Source: CAD feature listing. Evaluate the final solid. Frame: model axes, mm. Face numbers are marked on the shaded views. A direction names the side the tool comes from. Give positions to 0.01 mm unless a question says otherwise; leave off trailing zeros. Loops run counter-clockwise (first coordinate to the right, second up) from the corner with the lowest first, then second, coordinate; pieces in that order, holes last. Notation, with made-up numbers: (80.25, 10) -> (127.25, 10) arc R23 ccw to (127.25, 25) -> close; hole circle Ø2 at (37.5, -10). An arc over 180 degrees is marked (long way). Return JSON: item names as keys, results as strings. Group by question number.
(1) Cut plane A-A on x = -46. Return loops of the section in (y, z).
(2) Pin query (flat end, axial travel): pin 1 (6 mm diameter, centred on y = -50, z = 31, fed in from -X); pin 2 (4.5 mm diameter, centred on x = -46, y = -21.5, fed in from -Z); pin 3 (5 mm diameter, centred on x = -46, y = 15.7, fed in from -Z); pin 4 (1 mm diameter, centred on x = 95.5, z = 49, fed in from +Y). Return the tip coordinate at first contact, or that it passes through.
(3) Cut plane C-C on z = 63. Return loops of the section in (x, y).
(4) Cut plane B-B on y = 5.5. Return loops of the section in (x, z).
(5) Access query for the marked faces 1, 2 and 3. Directions: +Z, -Z, +X, -X, +Y, -Y. A direction counts if a zero-diameter tool reaches every point of the face in a straight line with its end or side. Return the directions, or none.
(6) Cut plane D-D on y = -52. Return loops of the section in (x, z) (3 decimals), then the cut area to 3 significant figures.
(7) Ray query, line 1 (Y direction, x = 0, z = 3.25); line 2 (Y direction, x = -32, z = 57); line 3 (X direction, y = -24, z = 35). Return the intervals inside material, ascending. Write a range as from..to.
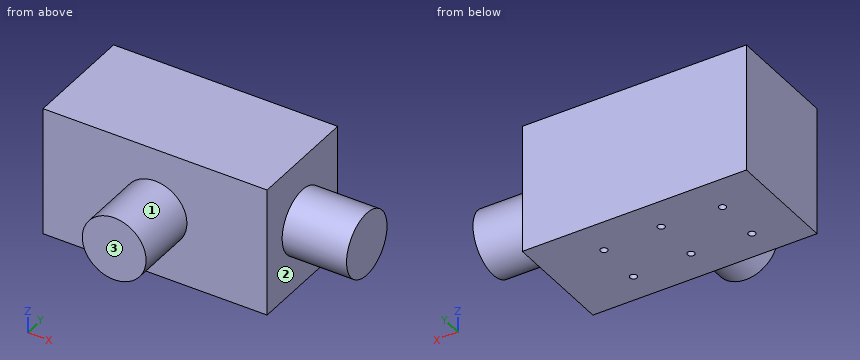
Autodesk Inventor part; units mm, degrees
ref_plane "YZ Plane" through (0, 0, 0) normal (1, 0, 0) x (0, 1, 0)
ref_plane "XZ Plane" through (0, 0, 0) normal (0, 1, 0) x (-1, 0, 0)
ref_plane "XY Plane" through (0, 0, 0) normal (0, 0, 1) x (1, 0, 0)
sketch "Sketch1" plane through (0, 0, 0) normal (0, 0, 1) x (1, 0, 0)
  line L0 (-13.5, 24) -> (13.5, 24) construction
  line L1 (13.5, 24) -> (13.5, -24) construction
  line L2 (13.5, -24) -> (-13.5, -24) construction
  line L3 (-13.5, -24) -> (-13.5, 24) construction
  line L4 (-13.5, 0) -> (13.5, 0) construction
  line L5 (0, -24) -> (0, 24) construction
  circle A0 centre (0, 18.3) radius 2.75
  circle A1 centre (0, -18.3) radius 2.75
  line L6 (-60, 21.2) -> (-32, 21.2) construction
  line L7 (-32, 21.2) -> (-32, -25.8) construction
  line L8 (-32, -25.8) -> (-60, -25.8) construction
  line L9 (-60, -25.8) -> (-60, 21.2) construction
  line L10 (-46, 21.2) -> (-46, -25.8) construction
  line L11 (-60, -2.3) -> (-32, -2.3) construction
  circle A2 centre (-46, 15.7) radius 2.75
  circle A3 centre (-46, -20.3) radius 2.75
  circle A4 centre (46, 15.7) radius 2.75
  circle A5 centre (46, -20.3) radius 2.75
  line L12 (-82, 43.2) -> (82, 43.2)
  line L13 (82, 43.2) -> (82, -43.2)
  line L14 (82, -43.2) -> (-82, -43.2)
  line L15 (-82, -43.2) -> (-82, 43.2)
  point P0 (0, 0)
  point P1 (0, 0)
  dimension "d0" = 27
  dimension "d1" = 48
  dimension "d2" = 5.5
  dimension "d3" = 36.6
  dimension "d4" = 28
  dimension "d5" = 47
  dimension "d7" = 2.3
  dimension "d8" = 46
  dimension "d9" = 5.5
  dimension "d10" = 36
  dimension "d11" = 22
  dimension "d19" = 43.2
extrude "Extrusion1" add sketch "Sketch1" along normal blind 10
sketch "Sketch3" plane through (0, 0, 10) normal (0, 0, 1) x (1, 0, 0)
  line L0 (-82, 43.2) -> (-82, -43.2)
  line L1 (-82, -43.2) -> (82, -43.2)
  line L2 (-82, 43.2) -> (82, 43.2)
  line L3 (82, 43.2) -> (82, -43.2)
  line L4 (82, -43.2) -> (-82, -43.2)
  line L5 (-82, -43.2) -> (-82, 43.2)
  point P0 (0, 0)
extrude "Extrusion3" add sketch "Sketch3" along normal blind 90
sketch "Sketch7" plane through (82, -43.2, 0) normal (1, 0, 0) x (0, 0, -1)
  line L0 (0, 0) -> (0, 86.4)
  line L1 (0, 86.4) -> (-100, 86.4)
  line L2 (-100, 0) -> (-100, 86.4)
  line L3 (0, 0) -> (-100, 0)
  point P0 (0, 43.2)
extrude "Extrusion7" add sketch "Sketch7" along normal blind 10
sketch "Sketch8" plane through (92, -43.2, 0) normal (1, 0, 0) x (0, 0, -1)
  line L0 (-100, 86.4) -> (-100, 0) construction
  line L1 (-100, 43.2) -> (0, 43.2) construction
  line L2 (0, 86.4) -> (-100, 86.4) construction
  line L3 (-50, 86.4) -> (-50, 0) construction
  circle A0 centre (-50, 43.2) radius 24.765
  dimension "d30" = 49.53
extrude "Extrusion8" add sketch "Sketch8" along normal blind 50
sketch "Sketch9" plane through (-82, -43.2, 0) normal (0, -1, 0) x (1, 0, 0)
  line L0 (174, 100) -> (174, 0) construction
  line L1 (174, 50) -> (0, 50) construction
  line L2 (0, 0) -> (0, 100) construction
  line L3 (0, 0) -> (174, 0) construction
  line L4 (87, 0) -> (87, 100) construction
  line L5 (0, 100) -> (174, 100) construction
  circle A0 centre (87, 50) radius 24.765
  point P0 (82, 0)
  dimension "d33" = 49.53
extrude "Extrusion9" add sketch "Sketch9" along normal blind 50
properties part number "aux_L"
Answers:
{
 "1": {"outline": "(-43.2, 0) -> (-23.05, 0) -> (-23.05, 10) -> (-17.55, 10) -> (-17.55, 0) -> (12.95, 0) -> (12.95, 10) -> (18.45, 10) -> (18.45, 0) -> (43.2, 0) -> (43.2, 100) -> (-43.2, 100) -> close"},
 "2": {"pin 1": "x = -13.9", "pin 2": "z = 0", "pin 3": "z = 10", "pin 4": "y = 24.76"},
 "3": {"outline": "(-82, -43.2) -> (-16.08, -43.2) -> (-16.08, -93.2) -> (26.08, -93.2) -> (26.08, -43.2) -> (92, -43.2) -> (92, -21.08) -> (142, -21.08) -> (142, 21.08) -> (92, 21.08) -> (92, 43.2) -> (-82, 43.2) -> close"},
 "4": {"outline": "(-82, 0) -> (92, 0) -> (92, 25.85) -> (142, 25.85) -> (142, 74.15) -> (92, 74.15) -> (92, 100) -> (-82, 100) -> close"},
 "5": {"face 1": "-Y", "face 2": "+X", "face 3": "+Z, -Z, +X, -X, -Y"},
 "6": {"outline": "circle Ø49.53 at (5, 50)", "area": "1,930 mm²"},
 "7": {"line 1": "-43.2..-21.05, -15.55..15.55, 21.05..43.2", "line 2": "-43.2..43.2", "line 3": "-82..92"}
}
